Geometry: see drawing. Coordinates: mm, zero at the bounding-box minimum. Give positions to 0.01 mm unless a question says otherwise; leave off trailing zeros. Loops run counter-clockwise (first coordinate to the right, second up) from the corner with the lowest first, then second, coordinate; pieces in that order, holes last. Notation, with made-up numbers: (64, 23.25) - (111, 23.25) arc R18 cw to (111, 41.25) - close; hole circle Ø6 at (-21.5, 11.25). An arc over 180 degrees is marked (long way). Use CSV: the item, a comma, the result in double quotes. Start each with the question number.
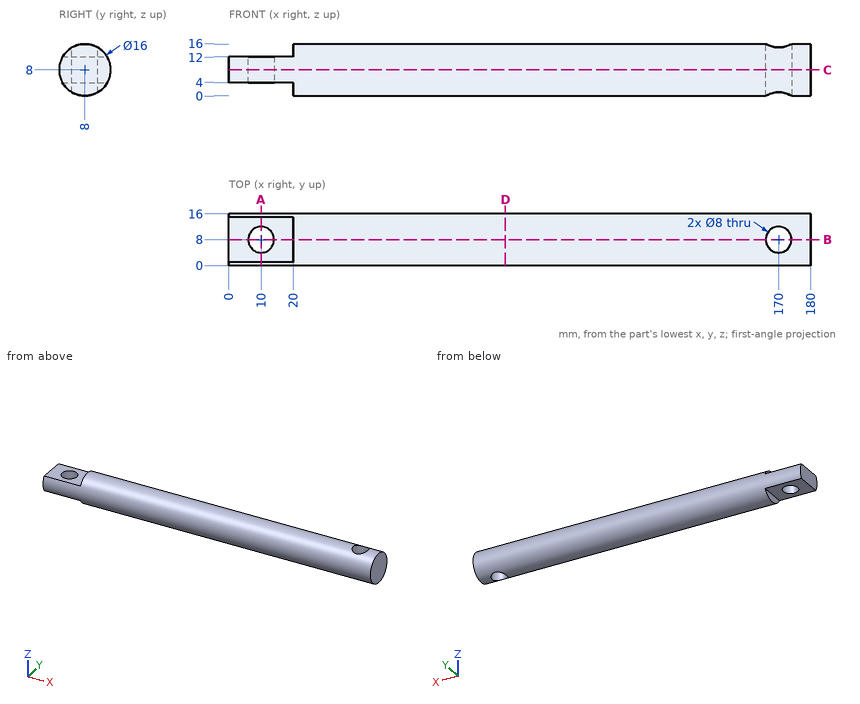
Item 1: Ray query, probe 1 along Y at (x, z) = (10, 8.75); probe 2 along Z at (x, y) = (73.5, 8.5); probe 3 along X at (y, z) = (5.5, 7.5). Return the intervals inside material, ascending.
Item 2: Section A-A (x = 10). Output: boundary loops of the cut face in (y, z), plus the area to 3 significant figures.
Item 3: Section C-C (z = 8). Output: boundary loops of the cut face in (x, y).
Item 4: Pin query (flat end, axial travel): pin 1 Ø5 at (x, z) = (131, 12.5) entering from -Y; pin 2 Ø2 at (y, z) = (9.5, 2.5) entering from -X; pin 3 Ø7 at (x, y) = (5.5, 6) entering from -Z. Return the tip coordinate at first contact, or that it passes through.
Item 5: Section B-B (y = 8). Output: boundary loops of the cut face in (x, z), plus the area to 3 significant figures.
Item 6: Section D-D (x = 85.5). Output: boundary loops of the cut face in (y, z).
Outcome:
1,probe 1,"y = 0.04 to 4, 12 to 15.96"
1,probe 2,"z = 0.02 to 15.98"
1,probe 3,"x = 0 to 6.88, 13.12 to 166.88, 173.12 to 180"
2,outline,"(1.07, 4) - (4, 4) - (4, 12) - (1.07, 12) arc R8 ccw to start; (12, 4) - (14.93, 4) arc R8 ccw to (14.93, 12) - (12, 12) - close"
2,area,"58.4 mm2"
3,outline,"(0, 0) - (180, 0) - (180, 16) - (0, 16) - close; hole circle Ø8 at (10, 8); hole circle Ø8 at (170, 8)"
4,pin 1,"stops at y = 0.25"
4,pin 2,"stops at x = 20"
4,pin 3,"stops at z = 4"
5,outline,"(0, 4) - (6, 4) - (6, 12) - (0, 12) - close; (14, 4) - (20, 4) - (20, 0) - (166, 0) - (166, 16) - (20, 16) - (20, 12) - (14, 12) - close; (174, 0) - (180, 0) - (180, 16) - (174, 16) - close"
5,area,"2,530 mm2"
6,outline,"circle Ø16 at (8, 8)"
